```python
from build123d import *

# Parameters (mm, degrees)
SKETCH1_R               = 24.97201
SKETCH1_R_2             = 21.79701
BOSS_EXTRUDE1_DEPTH     = 1047.75
SKETCH2_R               = 3.1115
CUT_EXTRUDE1_DEPTH      = 25.97201
SKETCH3_R               = 3.1115
CUT_EXTRUDE3_DEPTH      = 25.9720101
CUT_EXTRUDE3_DEPTH_BACK = 25.9720101


with BuildPart() as part:
    # Sketch1 → Boss-Extrude1 (new body)
    with BuildSketch(Plane(origin=(0, 0, 0), x_dir=(1, 0, 0), z_dir=(0, 1, 0))):
        Circle(SKETCH1_R)
        Circle(SKETCH1_R_2, mode=Mode.SUBTRACT)
    extrude(amount=BOSS_EXTRUDE1_DEPTH)

    # Sketch2 → Cut-Extrude1 (cut, symmetric)
    with BuildSketch(Plane(origin=(0, 0, 0), x_dir=(0, 0, -1), z_dir=(1, 0, 0))):
        with Locations((0, 12.7)):
            Circle(SKETCH2_R)
    cut_extrude1 = extrude(amount=CUT_EXTRUDE1_DEPTH, both=True, mode=Mode.SUBTRACT)

    # Mirror1: Cut-Extrude1 across plane
    add(cut_extrude1.mirror(Plane.ZX.offset(523.875)), mode=Mode.SUBTRACT)

    # Sketch3 → Cut-Extrude3 (cut, two sides)
    with BuildSketch(Plane(origin=(0, 0, 0), x_dir=(0, 0, -1), z_dir=(1, 0, 0))) as cut_extrude3_sk:
        with Locations((0, 933.45)):
            Circle(SKETCH3_R)
    extrude(amount=CUT_EXTRUDE3_DEPTH, mode=Mode.SUBTRACT)
    extrude(cut_extrude3_sk.sketch, amount=-CUT_EXTRUDE3_DEPTH_BACK, mode=Mode.SUBTRACT)


solid = part.part
```
Geometry check sheet. Reference: the model listing, model coordinates, mm. Coordinates: 2 decimals unless noted, no trailing zeros. Order: outer loops, then holes, each group sorted by start corner. A loop starts at its lowest first (then second) coordinate and runs counter-clockwise, first axis right, second up.
Item 1: Mould release check, pull along X, two halves, no side actions. Record for faces 1 (the cylindrical face through (20.79, 516.54, -6.55)), 2 (the flat face through (2, 0, -22)), 3 (the cylindrical face through (-3.25, 516.54, -24.76)): released by +X, released by -X, zero draft, split by the parting line, or undercut.
Item 2: Section check C-C (y = 812). Enter the section's corners in (x, z), plus the area to 4 significant figures.
Item 3: Section check B-B (z = -14). Enter the section's corners in (x, y), plus the area to 3 significant figures.
Item 4: Depth check by flat-ended pin: pin 1 (12 mm diameter, centred on x = -8.5, y = 546, fed in from -Z); pin 2 (1 mm diameter, centred on x = -6.5, y = 442, fed in from -Z); pin 3 (10 mm diameter, centred on y = 430, z = -19, fed in from +X). Enter the tip coordinate at first touch or a pass-through.
Item 5: Scan lines: line 1 along Y through (x, z) = (22.9, 0); line 2 along Z through (x, y) = (2, 459.5); line 3 along Z through (x, y) = (0, 674.5). Record each from-to range of solid material in increasing order.
Item 6: Section check A-A (x = 0). Enter the section's corners in (y, z), plus the area to 3 significant figures.
Check sheet entries:
1. face 1: undercut
1. face 2: zero draft
1. face 3: split by the parting line
2. outline: circle Ø49.94 at (0, 0); hole circle Ø43.59 at (0, 0)
2. area: 466.5 mm2
3. outline: (-20.68, 0) - (-16.71, 0) - (-16.71, 1047.75) - (-20.68, 1047.75) - close; (16.71, 0) - (20.68, 0) - (20.68, 1047.75) - (16.71, 1047.75) - close
3. area: 8,320 mm2
4. pin 1: stops at z = -24.85
4. pin 2: stops at z = -24.24
4. pin 3: stops at x = 20.68
5. line 1: y = 0 to 9.59, 15.81 to 930.34, 936.56 to 1031.94, 1038.16 to 1047.75
5. line 2: z = -24.89 to -21.71, 21.71 to 24.89
5. line 3: z = -24.97 to -21.8, 21.8 to 24.97
6. outline: (0, -24.97) - (1047.75, -24.97) - (1047.75, -21.8) - (0, -21.8) - close; (0, 21.8) - (1047.75, 21.8) - (1047.75, 24.97) - (0, 24.97) - close
6. area: 6,650 mm2
